Here's how the part is built. I have some questions about the finished solid (model axes, mm). A direction names the side the tool comes from. Coordinates: 2 decimals unless noted, no trailing zeros. Loops run counter-clockwise (first coordinate to the right, second up) from the corner with the lowest first, then second, coordinate; pieces in that order, holes last. Notation, with made-up numbers: (25.5, 5.5) -> (46.5, 5.5) arc R24 cw to (46.5, 41.5) -> close; hole circle Ø8 at (15, -24). An arc over 180 degrees is marked (long way). Answer as a JSON object with one key per item and string values. Group by question number.
Q1. I want a section at D-D on y = -4.5. Write out the boundary of the cut face in (x, z), then the cut area to 3 significant figures.
Q2. On a 3-axis mill with a long thin cutter (end or side, diameter ignored), from which of +Z, -Z, +X, -X, +Y, -Y can I reach the whole of each face in a straight line? I mean faces 1 (the flat face through (-15, 0, 0.508)), 2 (the flat face through (15, 0, 0)), 3 (the flat face through (-12, -3.175, -1)), 4 (the flat face through (-12, 3.175, -1)). Say none if no direction works.
Q3. I want a section at B-B on y = 1.25. Write out the boundary of the cut face in (x, z).
Q4. I want a section at A-A on z = 1.05. Write out the boundary of the cut face in (x, y) (3 decimals).
Q5. I need wall thicknesses on line 1 (Y direction, x = 11, z = 0.3) (3 decimals); line 2 (X direction, y = 3, z = -2.2); line 3 (X direction, y = -4.75, z = -2.5). Which ranges of each line are inside material? Lowest first, please.
Q6. I want a section at C-C on x = -12.5. Write out the boundary of the cut face in (y, z) (3 decimals).
Q7. I'm going to push flat-ended pins straight in: pin 1 (2.5 mm diameter, centred on x = 13, z = -1.5, fed in from +Y) (3 decimals); pin 2 (0.8 mm diameter, centred on x = 15.5, y = 0.5, fed in from +Z); pin 3 (1 mm diameter, centred on x = -13, z = -1.5, fed in from -Y) (3 decimals). Where does each tip first touch, or does it pass through?
Solid Edge part; units mm, degrees
sketch "Sketch1" plane through (0, 0, 0) normal (0, 0, 1) x (1, 0, 0)
  line L0 (-11.43, -1.7526) -> (-11.43, 1.7526)
  line L1 (-11.43, 1.7526) -> (-16.51, 1.7526)
  line L2 (-16.51, 1.7526) -> (-16.51, -1.7526)
  line L3 (-16.51, -1.7526) -> (-11.43, -1.7526)
  line L4 (16.51, 1.7526) -> (11.43, 1.7526)
  line L5 (11.43, 1.7526) -> (11.43, -1.7526)
  line L6 (11.43, -1.7526) -> (16.51, -1.7526)
  line L7 (16.51, -1.7526) -> (16.51, 1.7526)
extrude "Protrusion1" add sketch "Sketch1" along normal blind 0.508
sketch "Sketch2" plane through (0, 0, -3.2512) normal (0, 0, 1) x (1, 0, 0)
  line L0 (-13.97, -3.175) -> (13.97, -3.175)
  line L1 (-13.97, 3.175) -> (-13.97, -3.175)
  line L2 (13.97, 3.175) -> (-13.97, 3.175)
  line L3 (-4.9236, 10.033) -> (4.9236, 10.033)
  arc A0 (4.9236, 10.033) -> (4.9236, -10.033) centre (0, 0) cw
  line L4 (13.97, -3.175) -> (13.97, 3.175)
  line L5 (-4.9236, -10.033) -> (4.9236, -10.033)
  arc A1 (-4.9236, -10.033) -> (-4.9236, 10.033) centre (0, 0) cw
  arc A2 (-4.9236, -10.033) -> (-4.9236, 10.033) centre (0, 0) cw construction
extrude "ExtrudedProtrusion_2" add sketch "Sketch2" along normal blind 5.08
Result set:
{
 "1": {"outline": "(-10.23, -3.25) -> (10.23, -3.25) -> (10.23, 1.83) -> (-10.23, 1.83) -> close", "area": "104 mm²"},
 "2": {"face 1": "+Z, -X, +Y, -Y", "face 2": "-Z, +X, +Y, -Y", "face 3": "+Z, -Z, -X, -Y", "face 4": "+Z, -Z, -X, +Y"},
 "3": {"outline": "(-16.51, 0) -> (-13.97, 0) -> (-13.97, -3.25) -> (13.97, -3.25) -> (13.97, 0) -> (16.51, 0) -> (16.51, 0.51) -> (13.97, 0.51) -> (13.97, 1.83) -> (-13.97, 1.83) -> (-13.97, 0.51) -> (-16.51, 0.51) -> close"},
 "4": {"outline": "(-13.97, -3.175) -> (-10.716, -3.175) arc R11.176 ccw to (-4.924, -10.033) -> (4.924, -10.033) arc R11.176 ccw to (10.716, -3.175) -> (13.97, -3.175) -> (13.97, 3.175) -> (10.716, 3.175) arc R11.176 ccw to (4.924, 10.033) -> (-4.924, 10.033) arc R11.176 ccw to (-10.716, 3.175) -> (-13.97, 3.175) -> close"},
 "5": {"line 1": "y = -3.175 to 3.175", "line 2": "x = -13.97 to 13.97", "line 3": "x = -10.12 to 10.12"},
 "6": {"outline": "(-3.175, -3.251) -> (3.175, -3.251) -> (3.175, 1.829) -> (-3.175, 1.829) -> close"},
 "7": {"pin 1": "stops at y = 3.175", "pin 2": "stops at z = 0.51", "pin 3": "stops at y = -3.175"}
}
